```python
from build123d import *

# Parameters (mm, degrees)
F0_R     = 15
F1_DEPTH = 75
F2_SIZE  = 15
F3_SIZE  = 15
F4_R     = 10
F5_DEPTH = 15
F6_R     = 4.721078
F6_R_2   = 5
F7_DEPTH = 15


with BuildPart() as f1:
    # F0 (on Right) → F1 (new body)
    with BuildSketch(Plane.YZ):
        with BuildLine():
            Line((-50, -30), (0, -30))
            ThreePointArc((0, -30), (21.213203, -21.213203), (30, 0))
            Line((30, 0), (30, 15))
            Line((30, 15), (70, 15))
            Line((70, 15), (70, 30))
            Line((70, 30), (0, 30))
            ThreePointArc((0, 30), (-21.213203, 21.213203), (-30, 0))
            Line((-30, 0), (-30, -15))
            Line((-30, -15), (-40, -15))
            Line((-40, -15), (-40, 45))
            Line((-40, 45), (-50, 45))
            Line((-50, 45), (-50, 0))
            Line((-50, 0), (-50, -30))
        make_face()
        Circle(F0_R, mode=Mode.SUBTRACT)
    extrude(amount=F1_DEPTH)

    # F2
    f2_edges = [f1.edges().sort_by_distance(p)[0] for p in [
        (75, -45, 45),
    ]]
    chamfer(f2_edges, length=F2_SIZE)

    # F3
    f3_edges = [f1.edges().sort_by_distance(p)[0] for p in [
        (0, -45, 45),
    ]]
    chamfer(f3_edges, length=F3_SIZE)

    # F4 (on face) → F5 (cut)
    with BuildSketch(Plane.XZ.offset(50)):
        with Locations((37.181303, 10)):
            Circle(F4_R)
    extrude(amount=-F5_DEPTH, mode=Mode.SUBTRACT)

    # F6 (on face) → F7 (cut)
    with BuildSketch(Plane.XY.offset(30)):
        with Locations((55, 55)):
            Circle(F6_R)
        with Locations((20, 55)):
            Circle(F6_R_2)
    extrude(amount=-F7_DEPTH, mode=Mode.SUBTRACT)


solid = f1.part
```
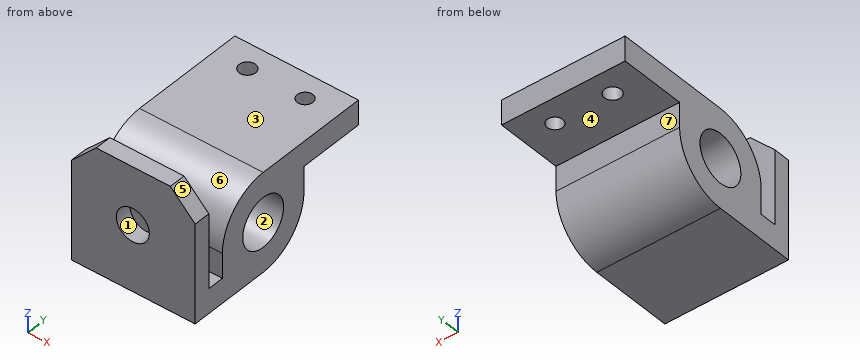
Model file for the job. Use its own axes, mm. Face numbers are marked on the shaded views. A direction names the side the tool comes from. Coordinates: 2 decimals unless noted, no trailing zeros. Loops run counter-clockwise (first coordinate to the right, second up) from the corner with the lowest first, then second, coordinate; pieces in that order, holes last. Notation, with made-up numbers: (-7, 58.5) -> (45, 58.5) arc R29 ccw to (45, 97.5) -> close; hole circle Ø4 at (-40, 81.5). An arc over 180 degrees is marked (long way). Answer as a JSON object with one key per item and string values.
Q1. Cut at C-C (x = 67.5). List the corners of the cut face in (y, z).
Report:
{"outline": "(-50, -30) -> (0, -30) arc R30 ccw to (30, 0) -> (30, 15) -> (70, 15) -> (70, 30) -> (0, 30) arc R30 ccw to (-30, 0) -> (-30, -15) -> (-40, -15) -> (-40, 37.5) -> (-50, 37.5) -> close; hole circle Ø30 at (0, 0)"}
Q2. 3-axis set-ups, long thin cutter, end or side, ignore diameter. For the marked faces 5, 6 and 7: which of +Z, -Z, +X, -X, +Y, -Y reach the whole face in a straight line?
Report:
{"face 5": "+Z, +X, +Y, -Y", "face 6": "+Z, +X, -X", "face 7": "-Z, +X, -X, +Y"}
Q3. Flat gauge pins, fed straight in: P1, Ø13, axis at x = 20, y = 55, coming from the -Z side; P2, Ø5.5, axis at x = 55, y = 55, coming from the +Z side; P3, Ø16.5, axis at x = 41.5, z = 5, coming from the +Y side; P4, Ø10, axis at x = 24, y = 18.5, coming from the -Z side. Where does each tip first touch, or does it go through?
Report:
{"P1": "stops at z = 15", "P2": "passes through", "P3": "stops at y = 30", "P4": "stops at z = -26.79"}
Q4. Probe probe 1 along Y at (x, z) = (20, 22); probe 2 along Y at (x, z) = (16.5, 18); probe 3 along Z at (x, y) = (44.5, 0). List the from-to ranges inside material, lowest first.
Report:
{"probe 1": "y = -50 to -40, -20.4 to 50, 60 to 70", "probe 2": "y = -50 to -40, -24 to 51.43, 58.57 to 70", "probe 3": "z = -30 to -15, 15 to 30"}
Q5. Cut at B-B (y = 55). List the corners of the cut face in (x, z).
Report:
{"outline": "(0, 15) -> (15, 15) -> (15, 30) -> (0, 30) -> close; (25, 15) -> (50.28, 15) -> (50.28, 30) -> (25, 30) -> close; (59.72, 15) -> (75, 15) -> (75, 30) -> (59.72, 30) -> close"}
Q6. Cut at A-A (x = 55). List the corners of the cut face in (y, z).
Report:
{"outline": "(-50, -30) -> (0, -30) arc R30 ccw to (30, 0) -> (30, 15) -> (50.28, 15) -> (50.28, 30) -> (0, 30) arc R30 ccw to (-30, 0) -> (-30, -15) -> (-40, -15) -> (-40, 45) -> (-50, 45) -> close; (59.72, 15) -> (70, 15) -> (70, 30) -> (59.72, 30) -> close; hole circle Ø30 at (0, 0)"}
Q7. Pull direction Z, two halves, no side cores. Call the marked faces 1, 2, 3 and 4: released by +Z, released by -Z, zero draft, split by the parting line, or undercut.
Report:
{"face 1": "undercut", "face 2": "undercut", "face 3": "released by +Z", "face 4": "released by -Z"}
Q8. Cut at D-D (z = 17). List the corners of the cut face in (x, y).
Report:
{"outline": "(0, -50) -> (30.04, -50) -> (30.04, -40) -> (0, -40) -> close; (0, -24.72) -> (75, -24.72) -> (75, 70) -> (0, 70) -> close; (44.32, -50) -> (75, -50) -> (75, -40) -> (44.32, -40) -> close; hole circle Ø10 at (20, 55); hole circle Ø9.44 at (55, 55)"}
